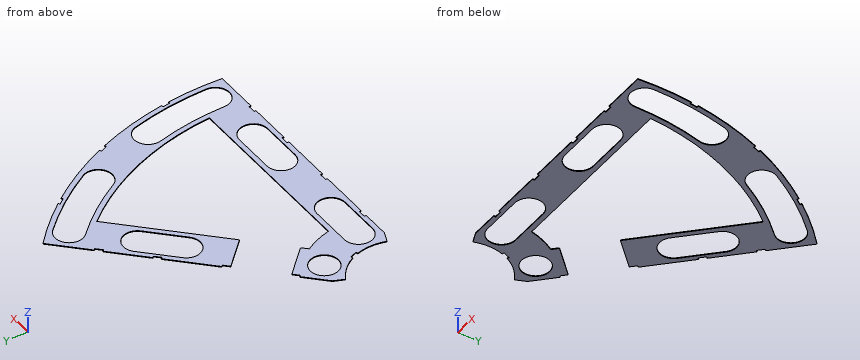
from build123d import *

# Parameters (mm, degrees)
BOSS_EXTRUDE1_DEPTH = 0.254
SKETCH2_R           = 4.699
CUT_EXTRUDE1_DEPTH  = 1.254
SKETCH3_W           = 2.54
SKETCH3_H           = 0.635
CUT_EXTRUDE2_DEPTH  = 1.254
CUT_EXTRUDE4_DEPTH  = 1.254
CUT_EXTRUDE5_DEPTH  = 1.254


with BuildPart() as part:
    # Sketch1 → Boss-Extrude1 (new body)
    with BuildSketch(Plane.XY):
        with BuildLine():
            Line((67.21146711, 76.191723231), (8.696654013, 17.676910134))
            Line((8.696654013, 17.676910134), (7.228954972, 14.133571205))
            ThreePointArc((7.228954972, 14.133571205), (14.666587579, 6.075099489), (15.105587123, -4.88230096))
            Line((15.105587123, -4.88230096), (18.648926052, -6.35))
            Line((18.648926052, -6.35), (101.401368334, -6.35))
            ThreePointArc((101.401368334, -6.35), (93.866160503, 38.880636728), (67.21146711, 76.191723231))
        make_face()
        with BuildLine():
            Line((88.672924278, 6.35), (27.86051193, 6.35))
            ThreePointArc((27.86051193, 6.35), (26.399857642, 10.93517908), (24.190484974, 15.210228852))
            Line((24.190484974, 15.210228852), (67.191354125, 58.211098004))
            ThreePointArc((67.191354125, 58.211098004), (82.13289044, 34.020557137), (88.672924278, 6.35))
        make_face(mode=Mode.SUBTRACT)
    extrude(amount=BOSS_EXTRUDE1_DEPTH)

    # Sketch2 → Cut-Extrude1 (cut, through all)
    with BuildSketch(Plane.XY.offset(0.254)):
        with Locations((22.225, 0)):
            Circle(SKETCH2_R)
        with Locations((36.195, 0)):
            Circle(SKETCH2_R)
        with Locations((61.722, 0)):
            Circle(SKETCH2_R)
        with Locations((75.692, 0)):
            Circle(SKETCH2_R)
        with Locations((95.25, 0)):
            Circle(SKETCH2_R)
        with Locations((15.715448212, 15.715448212)):
            Circle(SKETCH2_R)
        with Locations((25.593729945, 25.593729945)):
            Circle(SKETCH2_R)
        with Locations((43.644044748, 43.644044748)):
            Circle(SKETCH2_R)
        with Locations((53.522326482, 53.522326482)):
            Circle(SKETCH2_R)
        with Locations((92.004434954, 24.652514046)):
            Circle(SKETCH2_R)
        with Locations((82.48891971, 47.625)):
            Circle(SKETCH2_R)
        with Locations((67.351920908, 67.351920908)):
            Circle(SKETCH2_R)
    extrude(amount=-CUT_EXTRUDE1_DEPTH, mode=Mode.SUBTRACT)

    # Sketch3 → Cut-Extrude2 (cut, through all)
    with BuildSketch(Plane.XY.offset(0.254)):
        Polygon((15.266435406, 24.246691527), (17.06248663, 26.042742751), (17.511499436, 25.593729945), (15.715448212, 23.797678721), align=None)
        Polygon((44.991083167, 53.971339288), (43.195031942, 52.175288063), (43.644044748, 51.726275257), (45.440095973, 53.522326482), align=None)
        with Locations((29.21, -6.0325)):
            Rectangle(SKETCH3_W, SKETCH3_H)
        with Locations((68.707, -6.0325)):
            Rectangle(SKETCH3_W, SKETCH3_H)
        Polygon((29.230733674, 38.210989795), (31.026784898, 40.007041019), (31.475797704, 39.558028213), (29.67974648, 37.761976989), align=None)
        Polygon((56.845021246, 65.825277367), (55.048970022, 64.029226143), (55.497982828, 63.580213337), (57.294034052, 65.376264561), align=None)
        with Locations((48.9585, -6.0325)):
            Rectangle(SKETCH3_W, SKETCH3_H)
        with Locations((85.471, -6.0325)):
            Rectangle(SKETCH3_W, SKETCH3_H)
        Polygon((99.935462164, 14.437711971), (100.266998693, 11.919442024), (101.526133667, 12.085210288), (101.194597138, 14.603480236), align=None)
        Polygon((93.765504959, 37.464305742), (94.938831965, 37.950313702), (93.966816047, 40.296967714), (92.793489041, 39.810959755), align=None)
        Polygon((79.327792988, 62.471156422), (80.874047017, 60.456038938), (81.88160576, 61.229165953), (80.33535173, 63.244283437), align=None)
        Polygon((13.593916116, 7.005422516), (14.565932035, 4.658768503), (15.739259041, 5.144776462), (14.767243123, 7.491430475), align=None)
    extrude(amount=-CUT_EXTRUDE2_DEPTH, mode=Mode.SUBTRACT)

    # Sketch6 → Cut-Extrude4 (cut, through all)
    with BuildSketch(Plane.XY.offset(0.254)):
        with BuildLine():
            Line((40.321349984, 46.966739513), (50.199631717, 56.845021246))
            ThreePointArc((50.199631717, 56.845021246), (56.845021246, 56.845021246), (56.845021246, 50.199631717))
            Line((56.845021246, 50.199631717), (46.966739513, 40.321349984))
            ThreePointArc((46.966739513, 40.321349984), (40.321349984, 40.321349984), (40.321349984, 46.966739513))
        make_face()
        with BuildLine():
            Line((22.225, 4.699), (36.195, 4.699))
            ThreePointArc((36.195, 4.699), (40.894, 0), (36.195, -4.699))
            Line((36.195, -4.699), (22.225, -4.699))
            ThreePointArc((22.225, -4.699), (17.526, 0), (22.225, 4.699))
        make_face()
        with BuildLine():
            Line((61.722, 4.699), (75.692, 4.699))
            ThreePointArc((75.692, 4.699), (80.391, 0), (75.692, -4.699))
            Line((75.692, -4.699), (61.722, -4.699))
            ThreePointArc((61.722, -4.699), (57.023, 0), (61.722, 4.699))
        make_face()
        with BuildLine():
            ThreePointArc((99.949, 0), (99.093922449, 13.045962386), (96.543320412, 25.868704739))
            ThreePointArc((96.543320412, 25.868704739), (90.788244261, 29.191399504), (87.465549496, 23.436323353))
            ThreePointArc((87.465549496, 23.436323353), (89.776323642, 11.819277232), (90.551, 0))
            ThreePointArc((90.551, 0), (95.25, -4.699), (99.949, 0))
        make_face()
        with BuildLine():
            ThreePointArc((86.558373083, 49.9745), (79.294873009, 60.845096068), (70.674615673, 70.674615673))
            ThreePointArc((70.674615673, 70.674615673), (64.029226143, 70.674615673), (64.029226143, 64.029226143))
            ThreePointArc((64.029226143, 64.029226143), (71.838938317, 55.123956158), (78.419466338, 45.2755))
            ThreePointArc((78.419466338, 45.2755), (84.83841971, 43.555546628), (86.558373083, 49.9745))
        make_face()
    extrude(amount=-CUT_EXTRUDE4_DEPTH, mode=Mode.SUBTRACT)

    # Sketch5 → Cut-Extrude5 (cut, through all)
    with BuildSketch(Plane.XY.offset(0.254)):
        Polygon((14.278607232, 28.647017026), (26.626459399, 40.994869193), (40.994869193, 26.626459399), (28.647017026, 14.278607233), align=None)
    extrude(amount=-CUT_EXTRUDE5_DEPTH, mode=Mode.SUBTRACT)


solid = part.part
Read the model definition and answer for the solid it produces. Units are mm, in the model's axes. Round coordinates to 2 decimals unless told otherwise and drop trailing zeros. Write each loop counter-clockwise with the first axis right and the second up, starting at its lowest first coordinate (ties: lowest second). Pieces come first, ordered by that corner, then holes.
Q1. Find section B-B on z = 0.2. State how many separate pieces and enclosed holes the cut face has, and give its area (3 significant figures).
Values:
separate pieces: 1
enclosed holes: 6
area: 1,510 mm2
Q2. Straight lines are drawn through the part: line 1 (Y direction, x = 18, z = 0.1); line 2 (X direction, y = -1, z = 0.05); line 3 (Y direction, x = 60.5, z = 0.2). For each, find the intervals that lie inside material, in ascending order.
Values:
line 1: y = -6.08 to -2.06, 2.06 to 11.61, 19.82 to 24.93
line 2: x = 15.84 to 17.63, 40.79 to 57.13, 80.28 to 90.66, 99.84 to 101.6
line 3: y = -6.35 to -4.54, 4.54 to 6.35, 51.52 to 69.48
Q3. Find section A-A on y = 27.5. Determine the outline of the cut face in (x, z), and give its area (3 significant figures).
Values:
outline: (84.54, 0) - (88.27, 0) - (88.27, 0.25) - (84.54, 0.25) - close; (95.74, 0) - (97.81, 0) - (97.81, 0.25) - (95.74, 0.25) - close
area: 1.47 mm2
